from build123d import *

# Parameters (mm, degrees)
SKETCH1_R           = 101.6
BOSS_EXTRUDE1_DEPTH = 6.35
SKETCH2_R           = 25.4
CUT_EXTRUDE1_DEPTH  = 7.35
CUT_EXTRUDE2_DEPTH  = 7.35
CUT_EXTRUDE3_DEPTH  = 7.35
CUT_EXTRUDE10_DEPTH = 7.35


with BuildPart() as part:
    # Sketch1 → Boss-Extrude1 (new body)
    with BuildSketch(Plane.XY):
        Circle(SKETCH1_R)
    extrude(amount=BOSS_EXTRUDE1_DEPTH)

    # Sketch2 → Cut-Extrude1 (cut, through all)
    with BuildSketch(Plane.XY.offset(6.35)):
        Circle(SKETCH2_R)
    extrude(amount=-CUT_EXTRUDE1_DEPTH, mode=Mode.SUBTRACT)

    # Sketch3 → Cut-Extrude2 (cut, through all)
    with BuildSketch(Plane.XY.offset(6.35)):
        with BuildLine():
            ThreePointArc((69.838453591, 30.48), (0, 76.2), (-69.838453591, 30.48))
            ThreePointArc((-69.838453591, 30.48), (-63.278711326, 13.760257735), (-46.558969061, 20.32))
            ThreePointArc((-46.558969061, 20.32), (0, 50.8), (46.558969061, 20.32))
            ThreePointArc((46.558969061, 20.32), (63.278711326, 13.760257735), (69.838453591, 30.48))
        make_face()
    cut_extrude2 = extrude(amount=-CUT_EXTRUDE2_DEPTH, mode=Mode.SUBTRACT)

    # Mirror1: Cut-Extrude2 across plane
    add(cut_extrude2.mirror(Plane.ZX), mode=Mode.SUBTRACT)

    # Sketch4 → Cut-Extrude3 (cut, through all)
    with BuildSketch(Plane.XY.offset(6.35)):
        with BuildLine():
            Line((76.2, -3.175), (25.4, -3.175))
            ThreePointArc((25.4, -3.175), (22.225, 0), (25.4, 3.175))
            Line((25.4, 3.175), (76.2, 3.175))
            ThreePointArc((76.2, 3.175), (79.375, 0), (76.2, -3.175))
        make_face()
        with BuildLine():
            Line((-76.2, -3.175), (-25.4, -3.175))
            ThreePointArc((-25.4, -3.175), (-22.225, 0), (-25.4, 3.175))
            Line((-25.4, 3.175), (-76.2, 3.175))
            ThreePointArc((-76.2, 3.175), (-79.375, 0), (-76.2, -3.175))
        make_face()
    extrude(amount=-CUT_EXTRUDE3_DEPTH, mode=Mode.SUBTRACT)

    # Sketch14 → Cut-Extrude10 (cut, through all)
    with BuildSketch(Plane.XY.offset(6.35)):
        with BuildLine():
            Line((-58.198711326, -12.7), (-58.198711326, 12.7))
            ThreePointArc((-58.198711326, 12.7), (-51.242634846, 14.774417663), (-46.558969061, 20.32))
            ThreePointArc((-46.558969061, 20.32), (0, 50.8), (46.558969061, 20.32))
            ThreePointArc((46.558969061, 20.32), (51.242634846, 14.774417663), (58.198711326, 12.7))
            Line((58.198711326, 12.7), (58.198711326, -12.7))
            ThreePointArc((58.198711326, -12.7), (51.242634846, -14.774417663), (46.558969061, -20.32))
            ThreePointArc((46.558969061, -20.32), (0, -50.8), (-46.558969061, -20.32))
            ThreePointArc((-46.558969061, -20.32), (-51.242634846, -14.774417663), (-58.198711326, -12.7))
        make_face()
    extrude(amount=-CUT_EXTRUDE10_DEPTH, mode=Mode.SUBTRACT)


solid = part.part
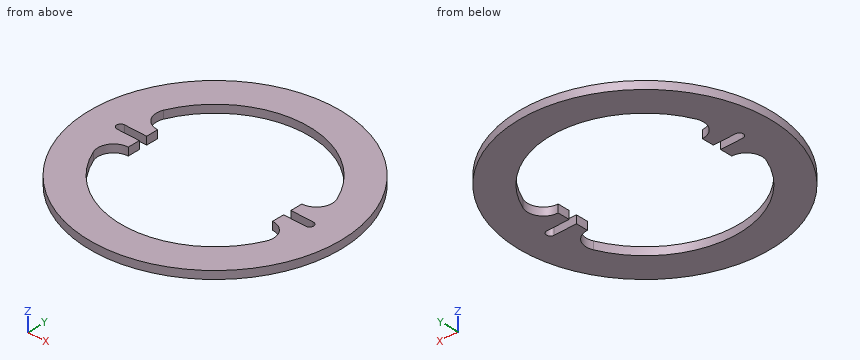
Can you work these out from the model? Positions are in its coordinate system, mm. Round coordinates to 2 decimals unless told otherwise and drop trailing zeros. Write each loop counter-clockwise with the first axis right and the second up, starting at its lowest first coordinate (ties: lowest second). Pieces come first, ordered by that corner, then holes. Notation, with made-up numbers: (59.5, 53.5) -> (108.5, 53.5) arc R24 ccw to (108.5, 92.5) -> close; hole circle Ø10 at (24, -29). An arc over 180 degrees is marked (long way). Use one line per item in the form item = value. Start each with the question number.
Q1. If I drill on probe 1 along Y at (x, z) = (-61, 4) (3 decimals); probe 2 along Y at (x, z) = (-2.5, 4.5); probe 3 along Y at (x, z) = (69.5, 3.25) (3 decimals), over which ranges is the centre line in solid material (lowest first)? Write a range as [from, to].
Q2. Imagine slicing it at B-B (x = 0). Please give me the cut outline in (y, z), then the cut area to 3 significant figures.
Q3. I'm going to push flat-ended pins straight in: P1, Ø1, axis at y = 23, z = 4, coming from the +X side; P2, Ø2, axis at x = -58, y = 14.5, coming from the +Z side; P3, Ø1, axis at x = 55, z = 3, coming from the -Y side; P4, Ø1.9, axis at x = -66, z = 2, coming from the -Y side. Where does each tip first touch, or does it pass through?
Q4. Imagine slicing it at C-C (z = 1.75). Please give me the cut outline in (x, y) (3 decimals), then the cut area to 3 significant figures.
Q5. Imagine slicing it at D-D (y = -86.5). Please give me the cut outline in (x, z), then the cut area to 3 significant figures.
Q6. Imagine slicing it at A-A (y = 0). Please give me the cut outline in (x, z) (3 decimals), then the cut area to 3 significant figures.
Worked out:
q1.probe_1 = [-81.25, -45.667], [-13.013, -3.175], [3.175, 13.013], [45.667, 81.25]
q1.probe_2 = [-101.57, -76.16], [76.16, 101.57]
q1.probe_3 = [-74.11, -31.244], [-19.606, -3.175], [3.175, 19.606], [31.244, 74.11]
q2.outline = (-101.6, 0) -> (-76.2, 0) -> (-76.2, 6.35) -> (-101.6, 6.35) -> close; (76.2, 0) -> (101.6, 0) -> (101.6, 6.35) -> (76.2, 6.35) -> close
q2.area = 323 mm^2
q3.P1 = 99.08
q3.P2 = through
q3.P3 = -85.75
q3.P4 = -78.05
q4.outline = circle Ø203.2 at (0, 0); hole (-76.2, -3.175) -> (-58.199, -3.175) -> (-58.199, -12.7) arc R12.7 ccw to (-69.838, -30.48) arc R76.2 ccw to (69.838, -30.48) arc R12.7 ccw to (58.199, -12.7) -> (58.199, -3.175) -> (76.2, -3.175) arc R3.175 ccw to (76.2, 3.175) -> (58.199, 3.175) -> (58.199, 12.7) arc R12.7 ccw to (69.838, 30.48) arc R76.2 ccw to (-69.838, 30.48) arc R12.7 ccw to (-58.199, 12.7) -> (-58.199, 3.175) -> (-76.2, 3.175) arc R3.175 ccw to start
q4.area = 15,100 mm^2
q5.outline = (-53.29, 0) -> (53.29, 0) -> (53.29, 6.35) -> (-53.29, 6.35) -> close
q5.area = 677 mm^2
q6.outline = (-101.6, 0) -> (-79.375, 0) -> (-79.375, 6.35) -> (-101.6, 6.35) -> close; (79.375, 0) -> (101.6, 0) -> (101.6, 6.35) -> (79.375, 6.35) -> close
q6.area = 282 mm^2
